from build123d import *

# Parameters (mm, degrees)
SKETCH1_W           = 55
SKETCH1_H           = 86
BOSS_EXTRUDE1_DEPTH = 3
SKETCH2_W           = 45
SKETCH2_H           = 45
CUT_EXTRUDE1_DEPTH  = 1.5
SKETCH3_W           = 61
SKETCH3_H           = 92
SKETCH3_W_2         = 55
SKETCH3_H_2         = 86
BOSS_EXTRUDE2_DEPTH = 70
SKETCH4_R           = 4.5
SKETCH4_R_2         = 2.5
CUT_EXTRUDE2_DEPTH  = 3
SKETCH5_R           = 4.5
CUT_EXTRUDE3_DEPTH  = 3


with BuildPart() as part:
    # Sketch1 → Boss-Extrude1 (new body)
    with BuildSketch(Plane(origin=(0, 0, 0), x_dir=(1, 0, 0), z_dir=(0, 1, 0))):
        Rectangle(SKETCH1_W, SKETCH1_H)
    extrude(amount=BOSS_EXTRUDE1_DEPTH)

    # Sketch2 → Cut-Extrude1 (cut)
    with BuildSketch(Plane(origin=(0, 3, 0), x_dir=(1, 0, 0), z_dir=(0, 1, 0))):
        Rectangle(SKETCH2_W, SKETCH2_H)
    extrude(amount=-CUT_EXTRUDE1_DEPTH, mode=Mode.SUBTRACT)

    # Sketch3 → Boss-Extrude2 (add)
    with BuildSketch(Plane(origin=(0, 0, 0), x_dir=(1, 0, 0), z_dir=(0, 1, 0))):
        Rectangle(SKETCH3_W, SKETCH3_H)
        Rectangle(SKETCH3_W_2, SKETCH3_H_2, mode=Mode.SUBTRACT)
    extrude(amount=BOSS_EXTRUDE2_DEPTH)

    # Sketch4 → Cut-Extrude2 (cut)
    with BuildSketch(Plane(origin=(30.5, 0, 0), x_dir=(0, 0, -1), z_dir=(1, 0, 0))):
        with Locations((-36, 48)):
            Circle(SKETCH4_R)
        with Locations((-12, 48)):
            Circle(SKETCH4_R)
        with Locations((12, 48)):
            Circle(SKETCH4_R)
        with Locations((36, 48)):
            Circle(SKETCH4_R)
        with Locations((36, 23)):
            Circle(SKETCH4_R)
        with Locations((12, 23)):
            Circle(SKETCH4_R)
        with Locations((-12, 23)):
            Circle(SKETCH4_R)
        with Locations((-36, 23)):
            Circle(SKETCH4_R)
        with Locations((-36, 33)):
            Circle(SKETCH4_R_2)
        with Locations((-12, 33)):
            Circle(SKETCH4_R_2)
        with Locations((12, 33)):
            Circle(SKETCH4_R_2)
        with Locations((36, 33)):
            Circle(SKETCH4_R_2)
        with Locations((36, 58)):
            Circle(SKETCH4_R_2)
        with Locations((12, 58)):
            Circle(SKETCH4_R_2)
        with Locations((-12, 58)):
            Circle(SKETCH4_R_2)
        with Locations((-36, 58)):
            Circle(SKETCH4_R_2)
    extrude(amount=-CUT_EXTRUDE2_DEPTH, mode=Mode.SUBTRACT)

    # Sketch5 → Cut-Extrude3 (cut)
    with BuildSketch(Plane(origin=(0, 0, -46), x_dir=(-1, 0, 0), z_dir=(0, 0, -1))):
        with Locations((19.818640834, 23)):
            Circle(SKETCH5_R)
        with Locations((19.818640834, 40)):
            Circle(SKETCH5_R)
        with Locations((19.818640834, 57)):
            Circle(SKETCH5_R)
    extrude(amount=-CUT_EXTRUDE3_DEPTH, mode=Mode.SUBTRACT)


solid = part.part
For this review, take the finished solid that the model builds, in its own axes (mm). A direction names the side the tool comes from. Round coordinates to 2 decimals unless told otherwise and drop trailing zeros. Loops run counter-clockwise (first coordinate to the right, second up) from the corner with the lowest first, then second, coordinate; pieces in that order, holes last. Notation, with made-up numbers: (4, -34.75) - (23, -34.75) arc R22 ccw to (23, -8.75) - close; hole circle Ø3 at (66.25, 52.5). An arc over 180 degrees is marked (long way). One line per item, written item: value. Start each with the question number.
Item 1: The part is to be moulded in two halves that separate along Y. For faces 1 (the flat face through (0, 0, -1)), 2 (the cylindrical face through (29, 58.1, 14.5)), 3 (the flat face through (0, 36, 43)), 4 (the flat face through (0, 1.5, 0)), say which applies: +Y half, -Y half, draft (parallel to the pull), parting line (faces both ways), or undercut.
Item 2: Take a section at A-A (z = -12). Give the boundary of the cut face in (x, y).
Item 3: Take a section at B-B (y = 23). Give the boundary of the cut face in (x, z).
Item 4: Clearance check with flat-ended pins moving along their axes: pin 1 Ø4 at (x, z) = (-22.5, 0) entering from +Y; pin 2 Ø13.5 at (x, z) = (3, 5.5) entering from +Y; pin 3 Ø4.5 at (y, z) = (33, -36) entering from +X. State where each tip first meets the part, or that it passes through.
Item 5: For faces 5 (the cylindrical face through (-16.5, 26.04, -44.52)), 6 (the cylindrical face through (29.021, 26.794, -14.419)), 7 (the flat face through (27.5, 36, 1)), 8 (the flat face through (30.5, 35, 1)), list the 3-axis set-ups (+Z, -Z, +X, -X, +Y, -Y) from which the entire face can be reached by the end or side of a thin tool; tool diameter is ignored.
Item 6: Take a section at D-D (x = 4.5). Give the boundary of the cut face in (y, z), plus the area to 4 significant figures.
Item 7: Take a section at C-C (y = 48). Give the boundary of the cut face in (x, z).
Item 8: For L1, parallel to Y at x = 29, z = -12; L2, parallel to X at y = 8.5, z = -11; L3, parallel to Z at x = -24, y = 32, list the stretches that pass through material, from the lowest coordinate up.
Answer below:
1. face 1: -Y half
1. face 2: undercut
1. face 3: draft
1. face 4: +Y half
2. outline: (-30.5, 0) - (30.5, 0) - (30.5, 18.5) - (27.5, 18.5) - (27.5, 3) - (22.5, 3) - (22.5, 1.5) - (-22.5, 1.5) - (-22.5, 3) - (-27.5, 3) - (-27.5, 70) - (-30.5, 70) - close; (27.5, 27.5) - (30.5, 27.5) - (30.5, 30.5) - (27.5, 30.5) - close; (27.5, 35.5) - (30.5, 35.5) - (30.5, 43.5) - (27.5, 43.5) - close; (27.5, 52.5) - (30.5, 52.5) - (30.5, 55.5) - (27.5, 55.5) - close; (27.5, 60.5) - (30.5, 60.5) - (30.5, 70) - (27.5, 70) - close
3. outline: (-30.5, -46) - (-24.32, -46) - (-24.32, -43) - (-27.5, -43) - (-27.5, 43) - (27.5, 43) - (27.5, 40.5) - (30.5, 40.5) - (30.5, 46) - (-30.5, 46) - close; (-15.32, -46) - (30.5, -46) - (30.5, -40.5) - (27.5, -40.5) - (27.5, -43) - (-15.32, -43) - close; (27.5, -31.5) - (30.5, -31.5) - (30.5, -16.5) - (27.5, -16.5) - close; (27.5, -7.5) - (30.5, -7.5) - (30.5, 7.5) - (27.5, 7.5) - close; (27.5, 16.5) - (30.5, 16.5) - (30.5, 31.5) - (27.5, 31.5) - close
4. pin 1: stops at y = 3
4. pin 2: stops at y = 1.5
4. pin 3: stops at x = -27.5
5. face 5: -Z
5. face 6: +X
5. face 7: +Y
5. face 8: +Z, -Z, +X, +Y, -Y
6. outline: (0, -46) - (70, -46) - (70, -43) - (3, -43) - (3, -22.5) - (1.5, -22.5) - (1.5, 22.5) - (3, 22.5) - (3, 43) - (70, 43) - (70, 46) - (0, 46) - close
6. area: 610.5 mm2
7. outline: (-30.5, -46) - (30.5, -46) - (30.5, -40.5) - (27.5, -40.5) - (27.5, -43) - (-27.5, -43) - (-27.5, 43) - (27.5, 43) - (27.5, 40.5) - (30.5, 40.5) - (30.5, 46) - (-30.5, 46) - close; (27.5, -31.5) - (30.5, -31.5) - (30.5, -16.5) - (27.5, -16.5) - close; (27.5, -7.5) - (30.5, -7.5) - (30.5, 7.5) - (27.5, 7.5) - close; (27.5, 16.5) - (30.5, 16.5) - (30.5, 31.5) - (27.5, 31.5) - close
8. L1: y = 0 to 18.5, 27.5 to 30.5, 35.5 to 43.5, 52.5 to 55.5, 60.5 to 70
8. L2: x = -30.5 to -27.5, 27.5 to 30.5
8. L3: z = -46 to -43, 43 to 46
